```python
from build123d import *

# Parameters (mm, degrees)
F0_W     = 86
F0_H     = 86
F1_DEPTH = 257
F2_R     = 10
F3_T     = -1


with BuildPart() as f1:
    # F0 (on Top) → F1 (new body)
    with BuildSketch(Plane.XY):
        Rectangle(F0_W, F0_H)
    extrude(amount=F1_DEPTH)

    # F2
    f2_edges = [f1.edges().sort_by_distance(p)[0] for p in [
        (43, 43, 128.5),
        (-43, -43, 128.5),
        (43, -43, 128.5),
        (-43, 43, 128.5),
    ]]
    fillet(f2_edges, radius=F2_R)

    # F3
    f3_openings = [f1.faces().sort_by_distance(p)[0] for p in [
        (0, 0, 257),
        (0, 0, 0),
    ]]
    offset(amount=F3_T, openings=f3_openings)


solid = f1.part
```
The model under review builds one solid part; all positions refer to its coordinate system, in mm. A direction names the side the tool comes from. Round coordinates to 2 decimals unless told otherwise and drop trailing zeros. Loops run counter-clockwise (first coordinate to the right, second up) from the corner with the lowest first, then second, coordinate; pieces in that order, holes last.
Item 1: Mouldability with a two-part tool opening along Y and no side actions: class faces 3 (the face through (-43, 0, 127)), 4 (the face through (0, 42, 127)), 5 (the face through (40.15, 39.99, 130.3)) as released by +Y, released by -Y, zero draft, split by the parting line, or undercut.
Determined:
face 3: zero draft
face 4: undercut
face 5: released by +Y
Item 2: Take a section at C-C (z = 17.5). Write out the cut boundary in (x, y).
Determined:
outline: (-43, -33) arc R10 ccw to (-33, -43) - (33, -43) arc R10 ccw to (43, -33) - (43, 33) arc R10 ccw to (33, 43) - (-33, 43) arc R10 ccw to (-43, 33) - close; hole (-42, -33) arc R9 ccw to (-33, -42) - (33, -42) arc R9 ccw to (42, -33) - (42, 33) arc R9 ccw to (33, 42) - (-33, 42) arc R9 ccw to (-42, 33) - close
Item 3: For faces 1 (the face through (0, -43, 127)), 2 (the face through (39.294, -39.434, 130.299)), list the 3-axis set-ups (+Z, -Z, +X, -X, +Y, -Y) from which the entire face can be reached by the end or side of a thin tool; tool diameter is ignored.
Determined:
face 1: +Z, -Z, +X, -X, -Y
face 2: +Z, -Z
Item 4: Take a section at A-A (y = -2). Write out the cut boundary in (x, z).
Determined:
outline: (-43, 0) - (-42, 0) - (-42, 257) - (-43, 257) - close; (42, 0) - (43, 0) - (43, 257) - (42, 257) - close
Item 5: For line 1 (X direction, y = 8.5, z = 120); line 2 (Y direction, x = -36.5, z = 54), list the stretches that pass through material, from the lowest coordinate up.
Determined:
line 1: x = -43 to -42, 42 to 43
line 2: y = -42.37 to -41.29, 41.29 to 42.37
